Here's the drawing with two shaded views (mm, measured from the low corner). I have some questions. Give positions to 0.01 mm unless a question says otherwise; leave off trailing zeros. Order: outer loops, then holes, each group sorted by start corner. A loop starts at its lowest first (then second) coordinate and runs counter-clockwise, first axis right, second up. Notation, with made-up numbers: M 61,31 L 110,31 A20 ccw 110,59 Z; hole C 33,-28 d5. An arc over 180 degrees is marked long. Write each question's results on one line, items separated by ' | '.
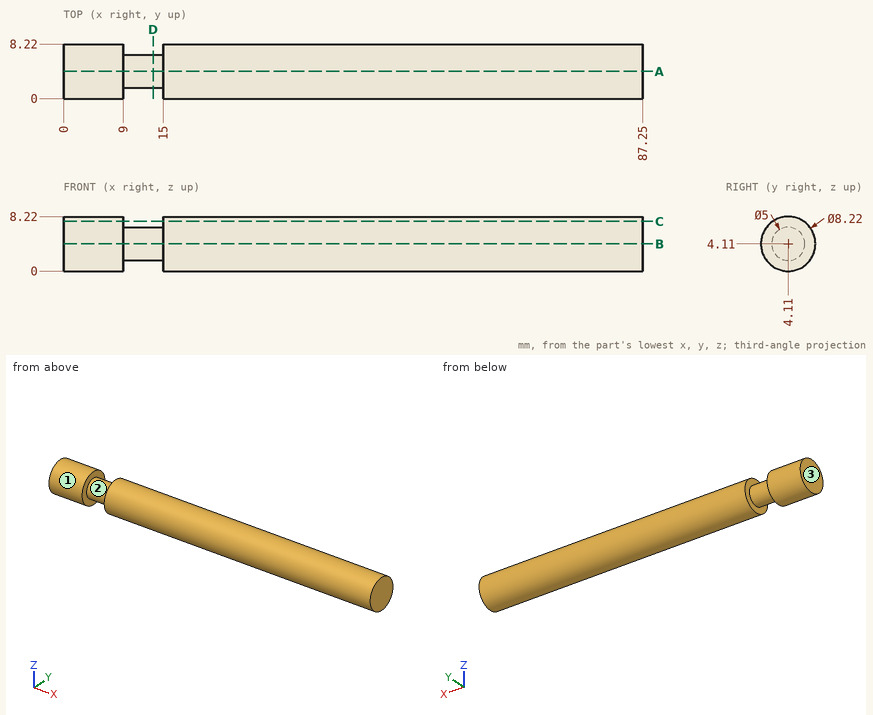
(1) Imagine slicing it at D-D, the plane x = 13.5. Write out the boundary of the cut face in (y, z).
Data:
outline: C 4.11,4.11 d5
(2) We'd pull the mould along X, two halves only. Please class the marked faces 1, 2 and 3: +X half, -X half, draft (parallel to the pull), parting line (faces both ways), or undercut.
Data:
face 1: draft | face 2: undercut | face 3: -X half
(3) Imagine slicing it at A-A, the plane y = 4.11. Write out the boundary of the cut face in (x, z), plus the area to 3 significant figures.
Data:
outline: M 0,0 L 9,0 L 9,1.61 L 15,1.61 L 15,0 L 87.25,0 L 87.25,8.22 L 15,8.22 L 15,6.61 L 9,6.61 L 9,8.22 L 0,8.22 Z | area: 698 mm2
(4) Will this pin go through, and if not, where does the flat tip stop? P1, Ø1.5, axis at x = 63.5, y = 1.5, coming from the +Z side.
Data:
P1: stops at z = 7.78
(5) I need wall thicknesses on L1, parallel to X at y = 4.5, z = 6.75; L2, parallel to Z at x = 24, y = 4.25; L3, parallel to Z at x = 65, y = 0.75. Which ranges of each line are inside material? Lowest first, please. Write a range as from..to.
Data:
L1: x = 0..9, 15..87.25 | L2: z = 0..8.22 | L3: z = 1.74..6.48
(6) Imagine slicing it at C-C, the plane z = 7.5. Write out the boundary of the cut face in (x, y).
Data:
outline: M 0,1.79 L 9,1.79 L 9,6.43 L 0,6.43 Z; M 15,1.79 L 87.25,1.79 L 87.25,6.43 L 15,6.43 Z
